Here's how the part is built. I have some questions about the finished solid (model axes, mm). Give positions to 0.01 mm unless a question says otherwise; leave off trailing zeros. Order: outer loops, then holes, each group sorted by start corner. A loop starts at its lowest first (then second) coordinate and runs counter-clockwise, first axis right, second up. Notation, with made-up numbers: M 2,78.25 L 30,78.25 A15 cw 30,85.25 Z; hole C 59,-5.75 d8. An arc over 180 degrees is marked long. Use one line per item in the form item = value.
from build123d import *

# Parameters (mm, degrees)
F0_W     = 3
F0_H     = 8
F0_W_2   = 23
F0_H_2   = 3
F1_DEPTH = 0.75
F2_DEPTH = 2.25
F3_DEPTH = 1.5


with BuildPart() as f1:
    # F0 (on Top) → F1 (new body)
    with BuildSketch(Plane.XY):
        with Locations((29, 0)):
            Rectangle(F0_W, F0_H)
        with Locations((-5.5, 5.5)):
            Rectangle(F0_W_2, F0_H_2)
        Polygon((-30.5, 4.013143), (-30.5, -4), (-27.5, -4), (-27.5, 4), (-27.5, 4.013143), align=None)
        with Locations((-5.5, -5.5)):
            Rectangle(F0_W_2, F0_H_2)
        Polygon((-30.5, 7), (-30.5, 4.013143), (-27.5, 4.013143), (-27.5, 4), (-17, 4), (-17, 7), align=None)
    extrude(amount=F1_DEPTH)

    # F0 (on Top) → F2 (join)
    with BuildSketch(Plane.XY):
        Polygon((-30.5, 4.013143), (-30.5, -4), (-27.5, -4), (-27.5, 4), (-27.5, 4.013143), align=None)
        with Locations((29, 0)):
            Rectangle(F0_W, F0_H)
    extrude(amount=F2_DEPTH)

    # F0 (on Top) → F3 (join)
    with BuildSketch(Plane.XY):
        Polygon((-30.5, 7), (-30.5, 4.013143), (-27.5, 4.013143), (-27.5, 4), (-17, 4), (-17, 7), align=None)
        Polygon((27.5, 4), (30.5, 4), (30.5, 7), (6, 7), (6, 4), align=None)
        Polygon((6, -7), (30.5, -7), (30.5, -4), (27.5, -4), (6, -4), align=None)
        Polygon((-30.5, -7), (-17, -7), (-17, -4), (-27.5, -4), (-30.5, -4), align=None)
        Polygon((-30.5, 4.013143), (-30.5, -4), (-27.5, -4), (-27.5, 4), (-27.5, 4.013143), align=None)
        with Locations((29, 0)):
            Rectangle(F0_W, F0_H)
    extrude(amount=F3_DEPTH)


solid = f1.part
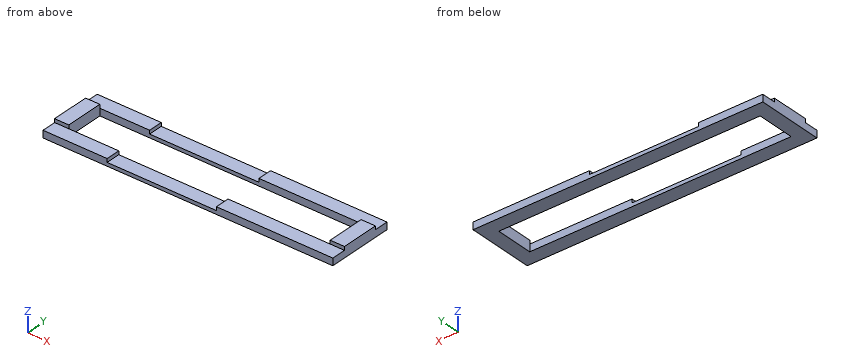
Q1. I want a section at A-A on x = -3.5. Write out the boundary of the cut face in (y, z), then the cut area to 3 significant figures.
Found:
outline = M -7,0 L -4,0 L -4,0.75 L -7,0.75 Z; M 4,0 L 7,0 L 7,0.75 L 4,0.75 Z
area = 4.50 mm²
Q2. I want a section at C-C on y = -5.25. Write out the boundary of the cut face in (x, z), then the cut area to 4 significant figures.
Found:
outline = M -30.5,0 L 30.5,0 L 30.5,1.5 L 6,1.5 L 6,0.75 L -17,0.75 L -17,1.5 L -30.5,1.5 Z
area = 74.25 mm²
Q3. I'm going to push flat-ended pins straight in: pin 1 Ø1.5 at (x, y) = (-25, 6) entering from +Z; pin 2 Ø0.6 at (x, z) = (28.5, 2) entering from -Y; pin 3 Ø1.5 at (x, y) = (-0.5, 6) entering from +Z. Where does each tip first touch, or does it pass through?
Found:
pin_1 = 1.5
pin_2 = -4
pin_3 = 0.75
Q4. I want a section at B-B on y = -2.25. Write out the boundary of the cut face in (x, z).
Found:
outline = M -30.5,0 L -27.5,0 L -27.5,2.25 L -30.5,2.25 Z; M 27.5,0 L 30.5,0 L 30.5,2.25 L 27.5,2.25 Z
Q5. I need wall thicknesses on L1, parallel to Y at x = 16, z = 1.3; L2, parallel to X at y = 2, z = 0.7; L3, parallel to X at y = -4.75, z = 0.9. Which ranges of each line are inside material? Lowest first, please.
Found:
L1 = -7 to -4, 4 to 7
L2 = -30.5 to -27.5, 27.5 to 30.5
L3 = -30.5 to -17, 6 to 30.5
